from build123d import *

# Parameters (mm, degrees)
SKETCH1_W           = 98
SKETCH1_H           = 42.5
BOSS_EXTRUDE1_DEPTH = 2
SKETCH2_W           = 13
SKETCH2_H           = 8
BOSS_EXTRUDE2_DEPTH = 35
SKETCH3_W           = 13
SKETCH3_H           = 28
BOSS_EXTRUDE3_DEPTH = 3


with BuildPart() as part:
    # Sketch1 → Boss-Extrude1 (new body)
    with BuildSketch(Plane(origin=(0, 0, 0), x_dir=(1, 0, 0), z_dir=(0, 1, 0))):
        Rectangle(SKETCH1_W, SKETCH1_H)
    extrude(amount=BOSS_EXTRUDE1_DEPTH)

    # Sketch2 → Boss-Extrude2 (add)
    with BuildSketch(Plane.XZ):
        Rectangle(SKETCH2_W, SKETCH2_H)
    extrude(amount=BOSS_EXTRUDE2_DEPTH)

    # Sketch3 → Boss-Extrude3 (add)
    with BuildSketch(Plane.XZ.offset(35)):
        Rectangle(SKETCH3_W, SKETCH3_H)
    extrude(amount=BOSS_EXTRUDE3_DEPTH)


solid = part.part
Read the model definition and answer for the solid it produces. Units are mm, in the model's axes. A direction names the side the tool comes from. Round coordinates to 2 decimals unless told otherwise and drop trailing zeros. Order: outer loops, then holes, each group sorted by start corner. A loop starts at its lowest first (then second) coordinate and runs counter-clockwise, first axis right, second up.
1) The part is cut by section A-A on z = -7. Write down the section's boundary in (x, y), plus the area to 3 significant figures.
2) The part is cut by section C-C on z = 17. Write down the section's boundary in (x, y).
3) Straight lines are drawn through the part: L1, parallel to Y at x = -1, z = -13.5; L2, parallel to Y at x = 24, z = -2; L3, parallel to Z at x = 4.5, y = -25. For each, find the intervals that lie inside material, in ascending order.
4) Flat-ended cylindrical pins translate along their axes: pin 1 (12 mm diameter, centred on x = 35.5, z = 15, fed in from -Y); pin 2 (3.5 mm diameter, centred on x = -0.5, y = -36, fed in from +Z); pin 3 (14 mm diameter, centred on y = -21.5, z = 1, fed in from -X). Find the tip coordinate at first contact, or state that the pin passes through.
5) For faces 1 (the face through (0, -17, -4)), 2 (the face through (0, -36, -14)), 3 (the face through (-6.5, -23, 0)), determine the directions among +Z, -Z, +X, -X, +Y, -Y from which every point of the face is accessible in a straight line to the end or side of a thin tool.
6) The mould has two halves that part along Y. Classify faces 4 (the face through (-1, 2, 0)), 5 (the face through (0, -38, 0)), 6 (the face through (0, -35, 9)), 7 (the face through (-1, 1, 21.25)): released by +Y, released by -Y, zero draft, split by the parting line, or undercut.
7) The part is cut by section B-B on y = -9. Write down the section's boundary in (x, z), plus the area to 3 significant figures.
Resolved:
1. outline: (-49, 0) - (49, 0) - (49, 2) - (-49, 2) - close; (-6.5, -38) - (6.5, -38) - (6.5, -35) - (-6.5, -35) - close
1. area: 235 mm2
2. outline: (-49, 0) - (49, 0) - (49, 2) - (-49, 2) - close
3. L1: y = -38 to -35, 0 to 2
3. L2: y = 0 to 2
3. L3: z = -4 to 4
4. pin 1: stops at y = 0
4. pin 2: stops at z = 14
4. pin 3: stops at x = -6.5
5. face 1: -Z, +X, -X
5. face 2: -Z, +X, -X, -Y
5. face 3: +Z, -Z, -X, -Y
6. face 4: released by +Y
6. face 5: released by -Y
6. face 6: undercut
6. face 7: zero draft
7. outline: (-6.5, -4) - (6.5, -4) - (6.5, 4) - (-6.5, 4) - close
7. area: 104 mm2
